from build123d import *

# Parameters (mm, degrees)
SKETCH2_W           = 6.7
SKETCH2_H           = 23.5
BOSS_EXTRUDE2_DEPTH = 0.8
CHAMFER1_SIZE       = 0.85
FILLET2_R           = 3.5
SKETCH6_R           = 1.4
CUT_EXTRUDE1_DEPTH  = 0.8


with BuildPart() as part:
    # Sketch2 → Boss-Extrude2 (new body)
    with BuildSketch(Plane(origin=(0, 0, 0), x_dir=(0, 0, -1), z_dir=(1, 0, 0))):
        Rectangle(SKETCH2_W, SKETCH2_H)
    extrude(amount=BOSS_EXTRUDE2_DEPTH)

    # Chamfer1
    # the kernel refuses this chamfer: 0.85 mm, written as the material it takes off along each edge
    with BuildSketch(Plane(origin=(0, -11.75, -5.53593054), x_dir=(0.9996219169112968, -0.02749587661058583, 0), z_dir=(0, 0, 1))) as chamfer1_piece_1:
        Polygon((CHAMFER1_SIZE * 0.999621916911, CHAMFER1_SIZE * 0.0274958766106), (-CHAMFER1_SIZE * 0.0274958766106, CHAMFER1_SIZE * 0.999621916911), (0, 0), align=None)
    extrude(amount=11.07186108, mode=Mode.SUBTRACT)

    # Fillet2
    # the kernel refuses this fillet: 3.5 mm, written as the material it takes off along each edge
    with BuildSketch(Plane(origin=(-8.75, 11.75, -3.35), x_dir=(0, -1, 0), z_dir=(1, 0, 0)), Plane(origin=(-8.75, 11.75, 3.35), x_dir=(0, 0, -1), z_dir=(1, 0, 0))) as fillet2_piece_1:
        with BuildLine():
            CenterArc((FILLET2_R, -FILLET2_R), FILLET2_R, 90, 90)
            Line((0, -FILLET2_R), (0, 0))
            Line((0, 0), (FILLET2_R, 0))
        make_face()
    extrude(amount=18.3, mode=Mode.SUBTRACT)

    # Sketch6 → Cut-Extrude1 (cut)
    with BuildSketch(Plane(origin=(0.8, 0, 0), x_dir=(0, 0, -1), z_dir=(1, 0, 0))):
        with Locations((-0.65, -0.3)):
            Circle(SKETCH6_R)
    extrude(amount=-CUT_EXTRUDE1_DEPTH, mode=Mode.SUBTRACT)


solid = part.part
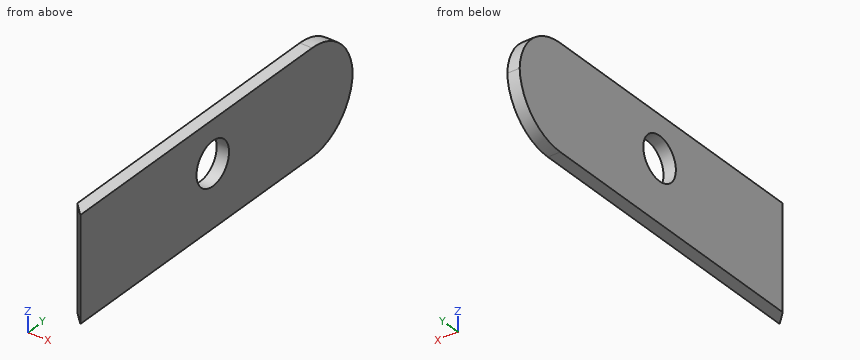
Verification items for the finished model (mm, model axes). Coordinates: 2 decimals unless noted, no trailing zeros. Loops run counter-clockwise (first coordinate to the right, second up) from the corner with the lowest first, then second, coordinate; pieces in that order, holes last. Notation, with made-up numbers: (53, 0.25) -> (60, 0.25) arc R10 cw to (60, 18.25) -> close; hole circle Ø9 at (14.25, -22). An arc over 180 degrees is marked (long way). Answer as CSV lines item,"result".
1) Cross-section at C-C, the plane z = 0.65. Record the cut outline in (x, y).
Found:
outline,"(0, -10.9) -> (0.8, -11.7) -> (0.8, -1.7) -> (0, -1.7) -> close; (0, 1.1) -> (0.8, 1.1) -> (0.8, 11.66) -> (0, 11.66) -> close"
2) Thickness scan on L1, parallel to Y at x = 0.5, z = 1.25; L2, parallel to Y at x = 0.4, z = 0.65; L3, parallel to Z at x = 0.35, y = 0.5. Record the ranges inside material, lowest first. Write a range as from..to.
Found:
L1,"y = -11.4..-1.56, 0.96..11.46"
L2,"y = -11.3..-1.7, 1.1..11.66"
L3,"z = -3.35..-0.5, 1.8..3.35"
3) Cross-section at A-A, the plane y = -0.3. Record the cut outline in (x, z).
Found:
outline,"(0, -3.35) -> (0.8, -3.35) -> (0.8, -0.75) -> (0, -0.75) -> close; (0, 2.05) -> (0.8, 2.05) -> (0.8, 3.35) -> (0, 3.35) -> close"
4) Cross-section at B-B, the plane x = 0.45. Record the cut outline in (y, z), then the cut area to 3 significant figures.
Found:
outline,"(-11.35, -3.35) -> (8.25, -3.35) arc R3.5 ccw to (11.75, 0) arc R3.5 ccw to (8.25, 3.35) -> (-11.35, 3.35) -> close; hole circle Ø2.8 at (-0.3, 0.65)"
area,"143 mm2"
5) Cross-section at D-D, the plane y = 10.5. Record the cut outline in (x, z), then the cut area to 3 significant figures.
Found:
outline,"(0, -2.53) -> (0.8, -2.53) -> (0.8, 2.53) -> (0, 2.53) -> close"
area,"4.05 mm2"
6) Depth check by flat-ended pin: pin 1 (3 mm diameter, centred on y = -0.3, z = 0.65, fed in from -X). Enter the tip coordinate at first touch or a pass-through.
Found:
pin 1,"stops at x = 0"
